Geometry check sheet. Reference: the model listing, model coordinates, mm. A direction names the side the tool comes from. Coordinates: 2 decimals unless noted, no trailing zeros. Order: outer loops, then holes, each group sorted by start corner. A loop starts at its lowest first (then second) coordinate and runs counter-clockwise, first axis right, second up. Notation, with made-up numbers: M -18,61 L 13,61 A28 ccw 13,85 Z; hole C 27.25,-6 d2. An arc over 180 degrees is marked long. Use CSV: the item, a comma, the result in double quotes. Start each with the question number.
```python
from build123d import *

# Parameters (mm, degrees)
BOSS_EXTRUDE1_DEPTH             = 80
BOSS_EXTRUDE2_REACH             = 99.687
SKETCH2_R                       = 6.375
SKETCH2_R_2                     = 4.9
BOSS_EXTRUDE2_DIRECTION_2_DEPTH = 570
F_6_0MM_DOWEL_HOLE1_D           = 6


with BuildPart() as part:
    # Sketch1 → Boss-Extrude1 (new body)
    with BuildSketch(Plane(origin=(0, 0, 0), x_dir=(0, 0, -1), z_dir=(1, 0, 0))):
        Polygon((0, 0), (25, 0), (25, -4), (4, -4), (4, -45), (0, -45), align=None)
    extrude(amount=BOSS_EXTRUDE1_DEPTH)

    # Boss-Extrude2: up to this plane
    boss_extrude2_end = Plane(origin=(80, -45, 0), z_dir=(0, 0, -1))
    # Sketch2 → Boss-Extrude2 (add, up to the surface)
    with BuildSketch(Plane(origin=(0, -39.220758573, 15.055438643), x_dir=(-1, 0, 0), z_dir=(0, 0.9335804264972002, -0.3583679495453042)), mode=Mode.PRIVATE) as boss_extrude2_sk1:
        with Locations(Location((-40, -8, 0), (0, 0, 90))):
            Circle(SKETCH2_R)
        with Locations(Location((-40, -8, 0), (0, 0, 90))):
            Circle(SKETCH2_R_2, mode=Mode.SUBTRACT)
    boss_extrude2_tool1 = split(extrude(boss_extrude2_sk1.sketch, amount=BOSS_EXTRUDE2_REACH, mode=Mode.PRIVATE), bisect_by=boss_extrude2_end, keep=Keep.BOTH, mode=Mode.PRIVATE)
    add(boss_extrude2_tool1.solids().sort_by_distance((40, -44.30768, 1.803556))[0])

    # Sketch2 → Boss-Extrude2 direction 2 (add)
    with BuildSketch(Plane(origin=(0, -39.220758573, 15.055438643), x_dir=(-1, 0, 0), z_dir=(0, 0.9335804264972002, -0.3583679495453042))):
        with Locations(Location((-40, -8, 0), (0, 0, 90))):
            Circle(SKETCH2_R)
        with Locations(Location((-40, -8, 0), (0, 0, 90))):
            Circle(SKETCH2_R_2, mode=Mode.SUBTRACT)
    extrude(amount=-BOSS_EXTRUDE2_DIRECTION_2_DEPTH)

    # 6.0mm Dowel Hole1 (through all)
    with Locations(Plane(origin=(0, 0, 0), x_dir=(1, 0, 0), z_dir=(0, 1, 0))):
        with Locations((25, 14.5), (55, 14.5)):
            Hole(F_6_0MM_DOWEL_HOLE1_D / 2)


solid = part.part
```
1) Draft check along Y on faces 1 (the face through (40, -23, 0)), 2 (the face through (39, 0, -12)), 3 (the face through (80, -16, -3)). Enter one of: +Y half, -Y half, draft (parallel to the pull), parting line (faces both ways), or undercut.
2) Section check A-A on x = 71. Record the boundary of the cut face in (y, z).
3) Gauge pin test, flat ends, axial feed: P1, Ø12.5, axis at x = 29.5, y = -30.5, coming from the -Z side; P2, Ø13.5, axis at x = 50, y = -13, coming from the +Z side; P3, Ø6.5, axis at x = 38.5, z = -13.5, coming from the -Y side; P4, Ø2, axis at x = 32.5, y = -473.5, coming from the +Z side. Record the tip position at first contact, or that the pin passes through.
4) Material ranges on line 1 along X through (y, z) = (-2.5, -14.5); line 2 along Z through (x, y) = (55, -3.05); line 3 along Z through (x, y) = (26.5, -43.5), recorded low to high.
5) Set-up check for faces 4 (the face through (39, -4, -15)), 5 (the face through (35.78, -573.224, 214.474)): record each of +Z, -Z, +X, -X, +Y, -Y from which the full face is reachable in a straight line by a thin tool's end or side.
Results are:
1,face 1,"undercut"
1,face 2,"+Y half"
1,face 3,"draft"
2,outline,"M -45,-4 L -4,-4 L -4,-25 L 0,-25 L 0,0 L -45,0 Z"
3,P1,"stops at z = -4"
3,P2,"stops at z = 2.93"
3,P3,"stops at y = -4"
3,P4,"passes through"
4,line 1,"x = 0 to 22, 28 to 52, 58 to 80"
4,line 2,"z = -25 to -17.5, -11.5 to 0"
4,line 3,"z = -4 to 0"
5,face 4,"-Z, +X, -X, -Y"
5,face 5,"+Z, +X, -X, -Y"
